Read the model definition and answer for the solid it produces. Units are mm, in the model's axes. A direction names the side the tool comes from. Coordinates: 2 decimals unless noted, no trailing zeros. Order: outer loops, then holes, each group sorted by start corner. A loop starts at its lowest first (then second) coordinate and runs counter-clockwise, first axis right, second up. Notation, with made-up numbers: M 19.25,-31.75 L 40.25,-31.75 A18 ccw 40.25,-7.75 Z; hole C 25,-16 d3. An arc over 180 degrees is marked long. Put each result on its own line as item: value.
from build123d import *

# Parameters (mm, degrees)
SKETCH001_R  = 40
PAD001_DEPTH = 90
SKETCH_R     = 50
PAD_DEPTH    = 100
CHAMFER_SIZE = 3


with BuildPart() as body001:
    # Sketch001 → Pad001 (new body)
    with BuildSketch(Plane.XY):
        Circle(SKETCH001_R)
    extrude(amount=PAD001_DEPTH)


with BuildPart() as chamfer_body:
    # Sketch → Pad (new body)
    with BuildSketch(Plane.XY):
        Circle(SKETCH_R)
    extrude(amount=PAD_DEPTH)

    # Cut: cut Body001
    add(body001.part, mode=Mode.SUBTRACT)

    # Chamfer
    chamfer_edges = [chamfer_body.edges().sort_by_distance(p)[0] for p in [
        (-40, 0, 0),
    ]]
    chamfer(chamfer_edges, length=CHAMFER_SIZE)


solid = chamfer_body.part
Q1. A tool of negligible diameter and unlimited length cuts with its end or side. For faces 4 (the face through (-1, 1, 90)), 5 (the face through (-1, 1, 100)), from which of +Z, -Z, +X, -X, +Y, -Y can it reach the whole face along a straight path? Write none if from no direction.
Answers below:
face 4: -Z
face 5: +Z, +X, -X, +Y, -Y
Q2. Given pin 1 (1.5 mm diameter, centred on y = 33.5, z = 54, fed in from -X); pin 2 (5 mm diameter, centred on x = -24, z = 66.5, fed in from -Y); pin 3 (3 mm diameter, centred on y = 14, z = 84, fed in from -X), each flat-ended and moving along its own axis, determine where each tip first touches the part or whether it passes through.
Answers below:
pin 1: stops at x = -37.78
pin 2: stops at y = -45.14
pin 3: stops at x = -48.41
Q3. Find section A-A on y = 0. Write down the section's boundary in (x, z), plus the area to 3 significant figures.
Answers below:
outline: M -50,0 L -43,0 L -40,3 L -40,90 L 40,90 L 40,3 L 43,0 L 50,0 L 50,100 L -50,100 Z
area: 2,790 mm^2
Q4. Consider line 1 along Y through (x, z) = (0, 37); line 2 along Z through (x, y) = (15, 31.5); line 3 along X through (y, z) = (-36.5, 68.5). Determine where each line is inside the solid, lowest interval first.
Answers below:
line 1: y = -50 to -40, 40 to 50
line 2: z = 90 to 100
line 3: x = -34.17 to -16.36, 16.36 to 34.17
Q5. For a pull along X with two mould halves and no side action, classify faces 1 (the face through (22, 37.3, 0)), 2 (the face through (47.69, 15.02, 49.3)), 3 (the face through (-8.67, -39.05, 45.89)) as +X half, -X half, draft (parallel to the pull), parting line (faces both ways), or undercut.
Answers below:
face 1: draft
face 2: parting line
face 3: undercut
Q6. Find section C-C on z = 79. Write down the section's boundary in (x, y).
Answers below:
outline: C 0,0 d100; hole C 0,0 d80
